Input: part model. Units: mm. Frame: model coordinates. A direction names the side the tool comes from. Round coordinates to 2 decimals unless told otherwise and drop trailing zeros. Write each loop counter-clockwise with the first axis right and the second up, starting at its lowest first coordinate (ties: lowest second). Pieces come first, ordered by that corner, then holes. Notation, with made-up numbers: (88.5, 55.25) -> (122.5, 55.25) arc R24 ccw to (122.5, 84.25) -> close; hole circle Ø5 at (0.5, 22.5). An arc over 180 degrees is marked (long way). Write item = value, one per line. Start each with the question number.
```python
from build123d import *

# Parameters (mm, degrees)
SKETCH_1_W          = 11
SKETCH_1_H          = 20
SKETCH_1_R          = 3.35
EXTRUDE_1_DEPTH     = 5
SKETCH_2_W          = 11
SKETCH_2_H          = 20
EXTRUDE_2_DEPTH     = 5
FILLET_1_R          = 5
FILLET_2_R          = 1
FILLET_4_R          = 1
FILLET_8_R          = 5
FILLET_9_R          = 5
CUT_EXTRUDE_3_DEPTH = 2
SKETCH_9_R          = 1.25
CUT_EXTRUDE_4_DEPTH = 3
FILLET_10_R         = 0.6


with BuildPart() as part:
    # Эскиз1 → Бобышка-Вытянуть1 (new body)
    with BuildSketch(Plane.XY):
        with Locations((0.5, 4.5)):
            Rectangle(SKETCH_1_W, SKETCH_1_H)
        Circle(SKETCH_1_R, mode=Mode.SUBTRACT)
    extrude(amount=EXTRUDE_1_DEPTH)

    # Эскиз2 → Бобышка-Вытянуть2 (add)
    with BuildSketch(Plane(origin=(0, 14.5, 0), x_dir=(1, 0, 0), z_dir=(0, 1, 0))):
        with Locations((0.5, 5)):
            Rectangle(SKETCH_2_W, SKETCH_2_H)
    extrude(amount=EXTRUDE_2_DEPTH)

    # Скругление1
    fillet_1_edges = [part.edges().sort_by_distance(p)[0] for p in [
        (0.5, 14.5, 0),
    ]]
    fillet(fillet_1_edges, radius=FILLET_1_R)

    # Скругление2
    fillet_2_edges = [part.edges().sort_by_distance(p)[0] for p in [
        (-3.35, 0, 0),
    ]]
    fillet(fillet_2_edges, radius=FILLET_2_R)

    # Скругление4
    fillet_4_edges = [part.edges().sort_by_distance(p)[0] for p in [
        (0.5, 19.5, 5),
    ]]
    fillet(fillet_4_edges, radius=FILLET_4_R)

    # Скругление8
    fillet_8_edges = [part.edges().sort_by_distance(p)[0] for p in [
        (6, -5.5, 2.5),
        (-5, -5.5, 2.5),
    ]]
    fillet(fillet_8_edges, radius=FILLET_8_R)

    # Скругление9
    fillet_9_edges = [part.edges().sort_by_distance(p)[0] for p in [
        (-5, 17, -15),
        (6, 17, -15),
    ]]
    fillet(fillet_9_edges, radius=FILLET_9_R)

    # Эскиз8 → Вырез-Вытянуть3 (cut)
    with BuildSketch(Plane.XZ.offset(-14.5)):
        Polygon((2.809401077, -9), (1.654700538, -7), (-0.654700538, -7), (-1.809401077, -9), (-0.654700538, -11), (1.654700538, -11), align=None)
    extrude(amount=-CUT_EXTRUDE_3_DEPTH, mode=Mode.SUBTRACT)

    # Эскиз9 → Вырез-Вытянуть4 (cut)
    with BuildSketch(Plane.XZ.offset(-16.5)):
        with Locations(Location((0.5, -9, 0), (0, 0, 270))):
            Circle(SKETCH_9_R)
    extrude(amount=-CUT_EXTRUDE_4_DEPTH, mode=Mode.SUBTRACT)

    # Скругление10
    fillet_10_edges = [part.edges().sort_by_distance(p)[0] for p in [
        (0.5, 19.5, -7.75),
    ]]
    fillet(fillet_10_edges, radius=FILLET_10_R)


solid = part.part
```
1. Section A-A (y = 0). Output: boundary loops of the cut face in (x, z).
2. Line query: line 1 along X through (y, z) = (18, -9); line 2 along Y through (x, z) = (0, 3.35); line 3 along Y through (x, z) = (4.5, -7.75). Output: solid intervals per line, ascending.
3. Reachability of faces 4 (the cylindrical face through (4.5, -4.07, 2.54)), 5 (the flat face through (0.4, 14.5, -11.2)), 6 (the flat face through (-1.224, 15.486, -7.986)) from +Z, -Z, +X, -X, +Y, -Y: full face, straight path, thin tool, end or side. Return the list, or none.
4. Mould query, pull axis X, two halves, no side actions, for faces 1 (the flat face through (0.5, -5.5, 2.5)), 2 (the flat face through (-5, 12, 1)), 3 (the flat face through (-1.24, 15.49, -9.99)). Classes: pulls with the +X half, pulls with the -X half, needs draft (parallel to the pull), parting line crosses it, or undercut.
5. Section C-C (z = -3.5). Output: boundary loops of the cut face in (x, y), then the cut area to 3 significant figures.
6. Section B-B (y = 12.25). Output: boundary loops of the cut face in (x, z), then the cut area to 3 significant figures.
7. Pin query (flat end, axial travel): P1, Ø1.5, axis at x = 4, z = -6, coming from the -Y side; P2, Ø10, axis at y = 4, z = -8, coming from the -X side; P3, Ø1.2, axis at x = 0, z = -10, coming from the -Y side. Return the tip coordinate at first contact, or that it passes through.
Check sheet entries:
q1.outline = (-5, 0) -> (-4.35, 0) arc R1 ccw to (-3.35, 1) -> (-3.35, 5) -> (-5, 5) -> close; (3.35, 1) arc R1 ccw to (4.35, 0) -> (6, 0) -> (6, 5) -> (3.35, 5) -> close
q2.line_1 = -5 to -0.75, 1.75 to 6
q2.line_2 = -5.5 to -3.35, 3.35 to 19.5
q2.line_3 = 14.5 to 19.5
q3.face_4 = +Z, -Z, +X, -Y
q3.face_5 = -Z, +X, -X, -Y
q3.face_6 = -Y
q4.face_1 = needs draft
q4.face_2 = pulls with the -X half
q4.face_3 = undercut
q5.outline = (-5, 14.27) -> (6, 14.27) -> (6, 19.5) -> (-5, 19.5) -> close
q5.area = 57.5 mm2
q6.outline = (-5, -0.82) -> (6, -0.82) -> (6, 5) -> (-5, 5) -> close
q6.area = 64.1 mm2
q7.P1 = 14.5
q7.P2 = through
q7.P3 = 16.5
